```python
from build123d import *

# Parameters (mm, degrees)
F0_W     = 19.05
F0_H     = 63.5
F1_DEPTH = 762
F2_SIZE  = 41.0464
F7_DEPTH = 19.051
F8_SIZE  = 22.45359


# Not quite as in the source:
# - a fillet or chamfer is up to 0.001 mm smaller than in the source, because OpenCascade refuses the exact size


with BuildPart() as f1:
    # F0 (on Front) → F1 (new body)
    with BuildSketch(Plane.XZ):
        with Locations((9.525, -31.75)):
            Rectangle(F0_W, F0_H)
    extrude(amount=F1_DEPTH)

    # F2
    f2_edges = [f1.edges().sort_by_distance(p)[0] for p in [
        (9.525, 0, 0),
        (9.525, -762, 0),
    ]]
    chamfer(f2_edges, length=F2_SIZE)

    # F6 (on face) → F7 (cut, through all)
    with BuildSketch(Plane(origin=(0, 0, 0), x_dir=(0, -1, 0), z_dir=(-1, 0, 0))):
        Polygon((0, -41.0493596973), (0, -63.5), (22.4506403027, -63.5), align=None)
    extrude(amount=-F7_DEPTH, mode=Mode.SUBTRACT)

    # F8 (size 22.4536 in the source; OpenCascade refuses exactly that, so slightly less here)
    f8_edges = [f1.edges().sort_by_distance(p)[0] for p in [
        (9.525, -762, -63.5),
    ]]
    chamfer(f8_edges, length=F8_SIZE)


solid = f1.part
```
CAD build for the part. Positions are in the model's coordinates, mm. Give positions to 0.01 mm unless a question says otherwise; leave off trailing zeros. Loops run counter-clockwise (first coordinate to the right, second up) from the corner with the lowest first, then second, coordinate; pieces in that order, holes last. Notation, with made-up numbers: (79.25, 13) - (132.25, 13) arc R19 cw to (132.25, 40) - close; hole circle Ø10 at (-3, 2.25). An arc over 180 degrees is marked (long way). Put each result on its own line as item: value.
Q1. Slice it at B-B (z = -34). Give the cut face in (x, y).
Filled in:
outline: (0, -754.95) - (19.05, -754.95) - (19.05, -7.05) - (0, -7.05) - close
Q2. Flat gauge pins, fed straight in: pin 1 (10 mm diameter, centred on x = 6.5, z = -16.5, fed in from +Y); pin 2 (8 mm diameter, centred on x = 7, z = -29.5, fed in from -Y); pin 3 (8 mm diameter, centred on x = 14, z = -57, fed in from -Y). Where does each tip first touch, or does it go through?
Filled in:
pin 1: stops at y = -19.55
pin 2: stops at y = -754.45
pin 3: stops at y = -750.05
Q3. Probe line 1 along Y through (x, z) = (5.25, -26); line 2 along Y through (x, z) = (9.5, -37). List the from-to ranges inside material, lowest first.
Filled in:
line 1: y = -746.95 to -15.05
line 2: y = -757.95 to -4.05
